Check sheet for the modelled part. Datum: model origin and axes. Units: mm. A direction names the side the tool comes from. Round coordinates to 2 decimals unless told otherwise and drop trailing zeros. Loops run counter-clockwise (first coordinate to the right, second up) from the corner with the lowest first, then second, coordinate; pieces in that order, holes last. Notation, with made-up numbers: M 71.5,47 L 120.5,47 A29 ccw 120.5,71 Z; hole C 28.5,24.25 d11. An arc over 180 degrees is marked long. One line per question, with ' | ' between items. Start each with the question number.
(1) Thickness scan on probe 1 along Z at (x, y) = (-6.5, 22.5); probe 2 along X at (y, z) = (0, -7.5). Record the ranges inside material, lowest first. Write a range as [from, to].
(2) Tool access check on faces 1 (the face through (-18.86, -10.8, -11.86)), 2 (the face through (10.94, 18.78, -11.86)), 3 (the face through (-21.733, 0, -12)). Record the directions out of +Z, -Z, +X, -X, +Y, -Y that give a thin tool (end or side, any length) a straight path to the whole face; none if there is none.
(3) Draft check along Z on faces 4 (the face through (0, -5, -24)), 5 (the face through (-1.5, 0.07, -11.83)), 6 (the face through (21.733, 0, -12)). Enter one of: +Z half, -Z half, draft (parallel to the pull), parting line (faces both ways), or undercut.
(4) Section check D-D (x = -13). Record the boundary of the cut face in (y, z), and give its area (3 significant figures).
(5) Go/stop test with flat-tipped pins: P1, Ø1.5, axis at y = 2.5, z = -15.5, coming from the -X side; P2, Ø6, axis at x = 3, z = -7.5, coming from the +Y side; P3, Ø12, axis at y = -10, z = -12, coming from the +X side. Record where each tip stops, or that it passes through.
(6) Section check A-A (y = 0). Record the boundary of the cut face in (x, z), and give its area (3 significant figures).
(7) Section check C-C (z = -11). Record the boundary of the cut face in (x, y).
Autodesk Fusion 360 part; units mm, degrees
sketch "Sketch1" plane through (0, 0, 0) normal (0, 0, 1) x (1, 0, 0)
  circle A0 centre (0, 0) radius 25
  circle A1 centre (0, 0) radius 22.5
  circle A2 centre (0, 0) radius 1.5
  line L0 (-0.912, -1.1909) -> (0.912, -1.1909)
  line L1 (5.8234, 21.7333) -> (-5.8234, 21.7333)
  line L2 (-5.8234, 21.7333) -> (-15.9099, 15.9099)
  line L3 (-15.9099, 15.9099) -> (-21.7333, 5.8234)
  line L4 (-21.7333, 5.8234) -> (-21.7333, -5.8234)
  line L5 (-21.7333, -5.8234) -> (-15.9099, -15.9099)
  line L6 (-15.9099, -15.9099) -> (-5.8234, -21.7333)
  line L7 (-5.8234, -21.7333) -> (5.8234, -21.7333)
  line L8 (5.8234, -21.7333) -> (15.9099, -15.9099)
  line L9 (15.9099, -15.9099) -> (21.7333, -5.8234)
  line L10 (21.7333, -5.8234) -> (21.7333, 5.8234)
  line L11 (21.7333, 5.8234) -> (15.9099, 15.9099)
  line L12 (15.9099, 15.9099) -> (5.8234, 21.7333)
  line L13 (1.75, 0) -> (22.5, 0)
  dimension "d2" = 50
  dimension "d3" = 45
  dimension "d4" = 3
  dimension "d5" = 1.824
  dimension "d38" = 2.5
  dimension "d42" = 22.5
extrude "Extrude6" add sketch "Sketch1" against normal blind 2 contours A0 | A1 L10 L13 | A1 L10 L13 | A1 L11 | L1 L2 L3 L4 L5 L6 L7 L8 L9 L10 L11 L12 | A1 L9 | A1 L12 | A1 L8 | A1 L1 | A1 L7 | A1 L2 | A1 L6 | A1 L3 | A1 L5 | A1 L4
extrude "Extrude7" add sketch "Sketch1" against normal blind 22 contours L1 L2 L3 L4 L5 L6 L7 L8 L9 L10 L11 L12
extrude "Extrude8" add sketch "Sketch1" along normal blind -24 and the other way blind 22 contours A0 | A1 L10 L13 | A1 L10 L13 | A1 L11 | L1 L2 L3 L4 L5 L6 L7 L8 L9 L10 L11 L12 | A1 L9 | A1 L12 | A1 L8 | A1 L1 | A1 L7 | A1 L2 | A1 L6 | A1 L3 | A1 L5 | A1 L4
equation "OuterDim = 50 mm"
equation "d2 = OuterDim"
equation "d3 = OuterDim * 0.9"
equation "Width = 20 mm"
equation "d42 = OuterDim * 0.9 / 2"
The answers:
1) probe 1: [-24, -22], [-2, 0] | probe 2: [-21.73, -1.5], [1.5, 21.73]
2) face 1: -X, -Y | face 2: +X, +Y | face 3: -X, +Y, -Y
3) face 4: -Z half | face 5: draft | face 6: undercut
4) outline: M -21.35,-24 L 21.35,-24 L 21.35,-22 L 17.59,-22 L 17.59,-2 L 21.35,-2 L 21.35,0 L -21.35,0 L -21.35,-2 L -17.59,-2 L -17.59,-22 L -21.35,-22 Z | area: 874 mm²
5) P1: x = -21.73 | P2: y = 21.73 | P3: x = 21.73
6) outline: M -25,-24 L -1.5,-24 L -1.5,0 L -25,0 L -25,-2 L -21.73,-2 L -21.73,-22 L -25,-22 Z; M 1.5,-24 L 25,-24 L 25,-22 L 21.73,-22 L 21.73,-2 L 25,-2 L 25,0 L 1.5,0 Z | area: 997 mm²
7) outline: M -21.73,-5.82 L -15.91,-15.91 L -5.82,-21.73 L 5.82,-21.73 L 15.91,-15.91 L 21.73,-5.82 L 21.73,5.82 L 15.91,15.91 L 5.82,21.73 L -5.82,21.73 L -15.91,15.91 L -21.73,5.82 Z; hole C 0,0 d3
